Read the model definition and answer for the solid it produces. Units are mm, in the model's axes. Face numbers are marked on the shaded views. A direction names the side the tool comes from. Coordinates: 2 decimals unless noted, no trailing zeros.
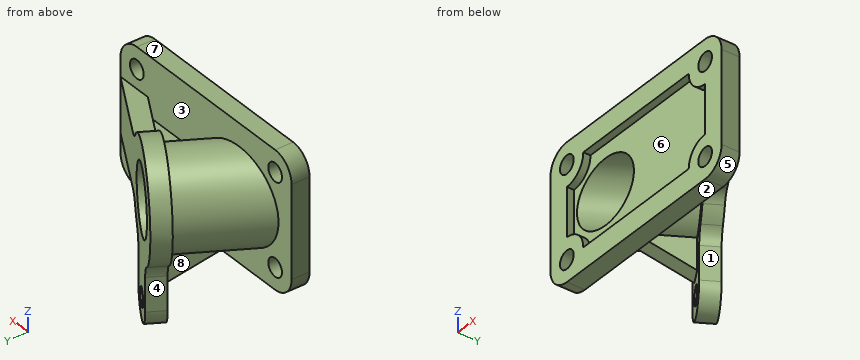
from build123d import *

# Parameters (mm, degrees)
SKETCH_7_R          = 5
EXTRUDE_5_DEPTH     = 10
CUT_EXTRUDE_3_DEPTH = 4
SKETCH_8_R          = 5
EXTRUDE_8_DEPTH     = 10
EXTRUDE_9_REACH     = 111.952
SKETCH_8_6_R        = 18
CUT_EXTRUDE_5_REACH = 111.952
SKETCH_8_7_R        = 18
RIB_9_REACH         = 119.31
SKETCH_10_WALL_W    = 268.526863554
SKETCH_10_WALL_H    = 10


with BuildPart() as part:
    # Sketch 7 → Extrude 5 (new body)
    # profile 1 of 2: a face of its own
    with BuildSketch(Plane(origin=(0, 0, 0), x_dir=(1, 0, 0), z_dir=(0, 1, 0))):
        with BuildLine():
            Line((-50.5, -37.5), (50.5, -37.5))
            ThreePointArc((50.5, -37.5), (58.985281374, -33.985281374), (62.5, -25.5))
            Line((62.5, -25.5), (62.5, 25.5))
            ThreePointArc((62.5, 25.5), (58.985281374, 33.985281374), (50.5, 37.5))
            Line((50.5, 37.5), (-50.5, 37.5))
            ThreePointArc((-50.5, 37.5), (-58.985281374, 33.985281374), (-62.5, 25.5))
            Line((-62.5, 25.5), (-62.5, -25.5))
            ThreePointArc((-62.5, -25.5), (-58.985281374, -33.985281374), (-50.5, -37.5))
        make_face()
        with Locations(Location((50.5, -25.5, 0), (0, 0, 270))):
            Circle(SKETCH_7_R, mode=Mode.SUBTRACT)
        with Locations(Location((-50.5, -25.5, 0), (0, 0, 270))):
            Circle(SKETCH_7_R, mode=Mode.SUBTRACT)
        with Locations(Location((50.5, 25.5, 0), (0, 0, 270))):
            Circle(SKETCH_7_R, mode=Mode.SUBTRACT)
        with Locations(Location((-50.5, 25.5, 0), (0, 0, 270))):
            Circle(SKETCH_7_R, mode=Mode.SUBTRACT)
        with BuildLine():
            Line((-38.5, 25.5), (38.5, 25.5))
            ThreePointArc((38.5, 25.5), (42.014718626, 17.014718626), (50.5, 13.5))
            Line((50.5, 13.5), (50.5, -13.5))
            ThreePointArc((50.5, -13.5), (42.014718626, -17.014718626), (38.5, -25.5))
            Line((38.5, -25.5), (-38.5, -25.5))
            ThreePointArc((-38.5, -25.5), (-42.014718626, -17.014718626), (-50.5, -13.5))
            Line((-50.5, -13.5), (-50.5, 13.5))
            ThreePointArc((-50.5, 13.5), (-42.014718626, 17.014718626), (-38.5, 25.5))
        make_face(mode=Mode.SUBTRACT)
    # profile 2 of 2: a face of its own
    with BuildSketch(Plane(origin=(0, 0, 0), x_dir=(1, 0, 0), z_dir=(0, 1, 0))):
        with BuildLine():
            ThreePointArc((38.5, 25.5), (42.014718626, 17.014718626), (50.5, 13.5))
            Line((50.5, 13.5), (50.5, -13.5))
            ThreePointArc((50.5, -13.5), (42.014718626, -17.014718626), (38.5, -25.5))
            Line((38.5, -25.5), (-38.5, -25.5))
            ThreePointArc((-38.5, -25.5), (-42.014718626, -17.014718626), (-50.5, -13.5))
            Line((-50.5, -13.5), (-50.5, 13.5))
            ThreePointArc((-50.5, 13.5), (-42.014718626, 17.014718626), (-38.5, 25.5))
            Line((-38.5, 25.5), (38.5, 25.5))
        make_face()
    extrude(amount=EXTRUDE_5_DEPTH)

    # Sketch 7_3 → Cut-Extrude 3 (cut)
    with BuildSketch(Plane(origin=(0, 0, 0), x_dir=(1, 0, 0), z_dir=(0, 1, 0))):
        with BuildLine():
            ThreePointArc((38.5, 25.5), (42.014718626, 17.014718626), (50.5, 13.5))
            Line((50.5, 13.5), (50.5, -13.5))
            ThreePointArc((50.5, -13.5), (42.014718626, -17.014718626), (38.5, -25.5))
            Line((38.5, -25.5), (-38.5, -25.5))
            ThreePointArc((-38.5, -25.5), (-42.014718626, -17.014718626), (-50.5, -13.5))
            Line((-50.5, -13.5), (-50.5, 13.5))
            ThreePointArc((-50.5, 13.5), (-42.014718626, 17.014718626), (-38.5, 25.5))
            Line((-38.5, 25.5), (38.5, 25.5))
        make_face()
    extrude(amount=CUT_EXTRUDE_3_DEPTH, mode=Mode.SUBTRACT)

    # Sketch 8 → Extrude 8 (add)
    with BuildSketch(Plane(origin=(19.955127019, 34.563293868, 0), x_dir=(0, 0, 1), z_dir=(0.500000000000001, 0.866025403784438, 0))):
        with BuildLine():
            Line((-5, 5.749364338), (-5, 49.126587737))
            Line((-5, 49.126587737), (-15, 49.126587737))
            Line((-15, 49.126587737), (-15, 5.351577729))
            ThreePointArc((-15, 5.351577729), (-15.986121811, 1.02145071), (-18.75, -2.454669769))
            ThreePointArc((-18.75, -2.454669769), (-22.173981002, -5.666617205), (-25.054939633, -9.373412263))
            ThreePointArc((-25.054939633, -9.373412263), (-28.663169687, -12.676820694), (-33.406586177, -13.873412263))
            Line((-33.406586177, -13.873412263), (-52, -13.873412263))
            ThreePointArc((-52, -13.873412263), (-64, -25.873412263), (-52, -37.873412263))
            Line((-52, -37.873412263), (-33.406586177, -37.873412263))
            ThreePointArc((-33.406586177, -37.873412263), (-28.663169687, -39.070003833), (-25.054939633, -42.373412263))
            ThreePointArc((-25.054939633, -42.373412263), (20.206795058, -48.047393266), (18.75, -2.454669769))
            ThreePointArc((18.75, -2.454669769), (15.986121811, 1.02145071), (15, 5.351577729))
            Line((15, 5.351577729), (15, 49.126587737))
            Line((15, 49.126587737), (5, 49.126587737))
            Line((5, 49.126587737), (5, 5.749364338))
            ThreePointArc((5, 5.749364338), (6.548457453, 0.4041395), (10.714285714, -3.285714691))
            ThreePointArc((10.714285714, -3.285714691), (0, -50.873412263), (-10.714285714, -3.285714691))
            ThreePointArc((-10.714285714, -3.285714691), (-6.548457453, 0.4041395), (-5, 5.749364338))
        make_face()
        with Locations(Location((-52, -25.873412263, 0), (0, 0, 270))):
            Circle(SKETCH_8_R, mode=Mode.SUBTRACT)
    extrude(amount=-EXTRUDE_8_DEPTH)

    # Sketch 8_6 → Extrude 9 (add, up to next)
    with BuildSketch(Plane(origin=(19.955127019, 34.563293868, 0), x_dir=(0, 0, 1), z_dir=(0.500000000000001, 0.866025403784438, 0)), mode=Mode.PRIVATE) as extrude_9_sk1:
        with BuildLine():
            Line((5, 49.126587737), (-5, 49.126587737))
            Line((-5, 49.126587737), (-5, 5.749364338))
            ThreePointArc((-5, 5.749364338), (-6.548457453, 0.4041395), (-10.714285714, -3.285714691))
            ThreePointArc((-10.714285714, -3.285714691), (0, -50.873412263), (10.714285714, -3.285714691))
            ThreePointArc((10.714285714, -3.285714691), (6.548457453, 0.4041395), (5, 5.749364338))
            Line((5, 5.749364338), (5, 49.126587737))
        make_face()
        with Locations(Location((0, -25.873412263, 0), (0, 0, 270))):
            Circle(SKETCH_8_6_R, mode=Mode.SUBTRACT)
    extrude_9_tool1 = extrude(extrude_9_sk1.sketch, amount=-EXTRUDE_9_REACH, mode=Mode.PRIVATE) - part.part
    add(extrude_9_tool1.solids().sort_by_distance((43.717111, 20.844306, 3.881966))[0])

    # Sketch 8_7 → Cut-Extrude 5 (cut, up to next)
    with BuildSketch(Plane(origin=(19.955127019, 34.563293868, 0), x_dir=(0, 0, 1), z_dir=(0.500000000000001, 0.866025403784438, 0)), mode=Mode.PRIVATE) as cut_extrude_5_sk1:
        with Locations(Location((0, -25.873412263, 0), (0, 0, 270))):
            Circle(SKETCH_8_7_R)
    cut_extrude_5_tool1 = extrude(cut_extrude_5_sk1.sketch, amount=-CUT_EXTRUDE_5_REACH, mode=Mode.PRIVATE) & part.part
    add(cut_extrude_5_tool1.solids().sort_by_distance((-2.451905, 47.5, 0))[0], mode=Mode.SUBTRACT)

    # Sketch 10 wall → Rib 9 (add, up to next)
    with BuildSketch(Plane(origin=(-14.201905284, 27.148403011, -33.5), x_dir=(-0.423116420047, -0.732859137032, 0.532813269688), z_dir=(0.266406634844, 0.461429827024, 0.846232840088)), mode=Mode.PRIVATE) as rib_9_sk1:
        Rectangle(SKETCH_10_WALL_W, SKETCH_10_WALL_H)
    rib_9_tool1 = extrude(rib_9_sk1.sketch, amount=RIB_9_REACH, mode=Mode.PRIVATE) - part.part
    add(rib_9_tool1.solids().sort_by_distance((-14.201905284, 27.148403011, -33.5))[0])


solid = part.part
Q1. Determine the mould class of the marked faces 5, 6, 7 and 8 for opening direction Z: +Z half, -Z half, draft (parallel to the pull), parting line (faces both ways), or undercut.
Findings below:
face 5: -Z half
face 6: undercut
face 7: +Z half
face 8: draft
Q2. A cutting plane is placed at A-A (y = 7). Count the separate pieces of the cut face and the enclosed holes in it, then the cut area to 3 significant figures.
Findings below:
separate pieces: 1
enclosed holes: 5
area: 7,760 mm2
Q3. Flat-ended cylindrical pins translate along their axes: pin 1 Ø2 at (x, z) = (26.5, -14) entering from +Y; pin 2 Ø1.5 at (x, z) = (-3, -23.5) entering from +Y; pin 3 Ø11.5 at (x, z) = (50.5, -25.5) entering from +Y. Find the tip coordinate at first contact, or state that the pin passes through.
Findings below:
pin 1: stops at y = 31.36
pin 2: stops at y = 48.25
pin 3: stops at y = 10
Q4. Which of the six approach directions +Z, -Z, +X, -X, +Y, -Y give full straight-line access (tool end or side, diameter ignored) to the marked faces 1, 2, 3 and 4?
Findings below:
face 1: -Z, +X
face 2: -Z, +X, -X, -Y
face 3: none
face 4: -Z, -X, +Y
Q5. Straight lines are drawn through the part: probe 1 along Z at (x, y) = (50, 5); probe 2 along X at (y, z) = (6, 25.5); probe 3 along X at (y, z) = (2, -25). For each, find the intervals that lie inside material, in ascending order.
Findings below:
probe 1: z = -37.5 to -30.47, -20.53 to 20.53, 30.47 to 37.5
probe 2: x = -62.5 to -55.5, -45.5 to 45.5, 55.5 to 62.5
probe 3: x = -62.5 to -55.47, -45.53 to -38.51, 38.51 to 45.53, 55.47 to 62.5
